Job drawing, mm, ordinate dimensions from the low corner. One solid piece. Give positions to 0.01 mm unless a question says otherwise; leave off trailing zeros. Write each loop counter-clockwise with the first axis right and the second up, starting at its lowest first coordinate (ties: lowest second). Pieces come first, ordered by that corner, then holes. Notation, with made-up numbers: M 74,-10 L 78,-10 A6 cw 78,-6 Z; hole C 12,-8 d6. An arc over 180 degrees is marked long. Use CSV: the item, a comma, the result in double quotes. Start each with the question number.
Item 1: Cut at A-A (x = 128). List the corners of the cut face in (y, z).
Item 2: Pin check, flat tips, straight feed: pin 1 (12 mm diameter, centred on x = 204.5, y = 51.5, fed in from +Z); pin 2 (1.5 mm diameter, centred on x = 120, y = 30, fed in from +Z) (1 decimal); pin 3 (12 mm diameter, centred on x = 187.5, y = 71.5, fed in from -Z) (1 decimal). Stop position of each tip, or through.
Item 3: Mould opens along Z. For the marked faces 1, 2, 3 and 4 say: released by +Z, released by -Z, zero draft, split by the parting line, or undercut.
Item 4: Cut at D-D (y = 69.5). List the corners of the cut face in (x, z).
Item 5: Cut at B-B (y = 49.5). List the corners of the cut face in (x, z).
Item 6: Cut at C-C (z = 128). List the corners of the cut face in (x, y).
Item 7: Drill centre lines: line 1 (Z direction, x = 217.5, y = 70.5) (1 decimal); line 2 (X direction, y = 70.5, z = 157.5); line 3 (X direction, y = 53.5, z = 117). Where is each one in solid material? Low to high. Write a range as [from, to].
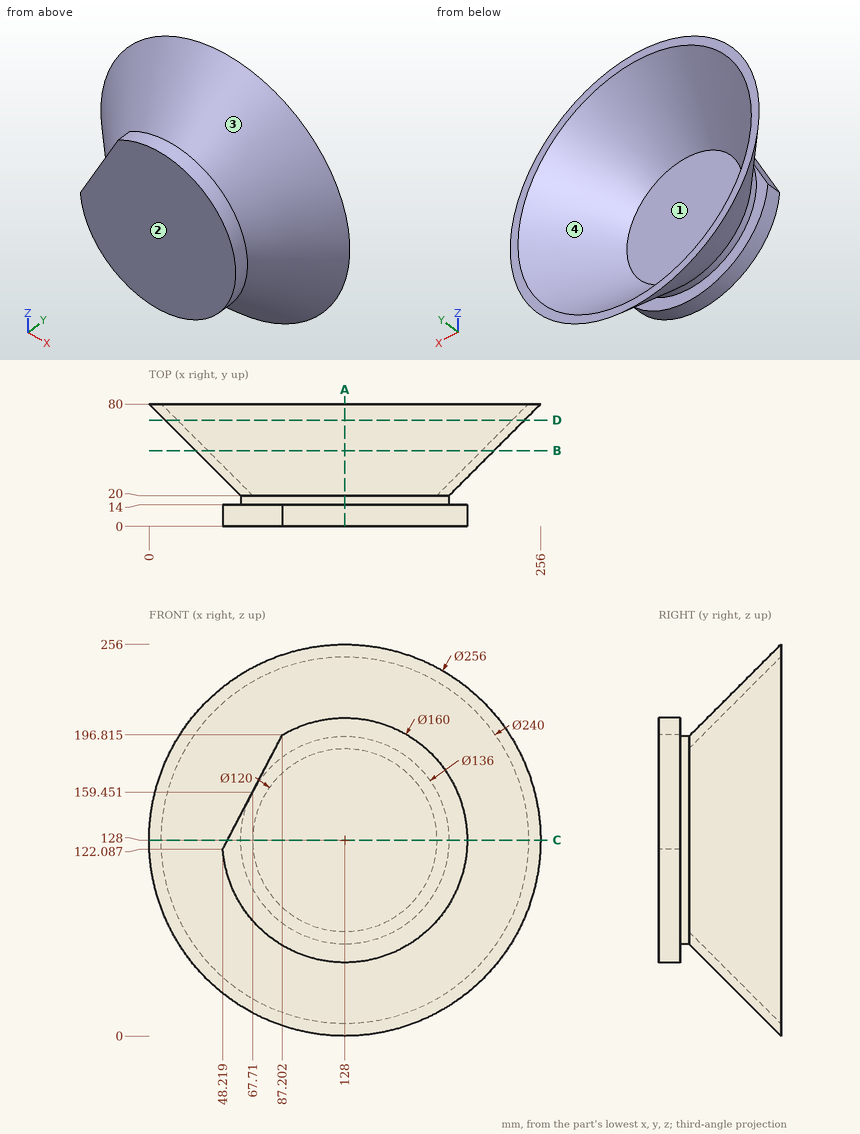
Worked answers:
1,outline,"M 0,48 L 14,48 L 14,60 L 20,60 L 80,0 L 80,8 L 20,68 L 20,188 L 80,248 L 80,256 L 20,196 L 14,196 L 14,208 L 0,208 Z"
2,pin 1,"stops at z = 202.6"
2,pin 2,"stops at z = 206.3"
2,pin 3,"stops at z = 16.8"
3,face 1,"undercut"
3,face 2,"zero draft"
3,face 3,"split by the parting line"
3,face 4,"undercut"
4,outline,"C 128,128 d235; hole C 128,128 d219"
5,outline,"C 128,128 d195; hole C 128,128 d179"
6,outline,"M 0,80 L 60,20 L 60,14 L 51.3,14 L 51.3,0 L 208,0 L 208,14 L 196,14 L 196,20 L 256,80 L 248,80 L 188,20 L 68,20 L 8,80 Z"
7,line 1,"z = [50.3, 63.2], [192.8, 205.7]"
7,line 2,"x = [13.23, 21.51], [234.49, 242.77]"
7,line 3,"x = [27.1, 35.15], [220.85, 228.9]"
